from build123d import *

# Parameters (mm, degrees)
SKETCH_1_R          = 3
EXTRUDE_1_DEPTH     = 5
EXTRUDE_1_2_DEPTH   = 5
EXTRUDE_1_3_DEPTH   = 5
EXTRUDE_1_4_DEPTH   = 5
SKETCH_2_R          = 30
EXTRUDE_2_DEPTH     = 5
SKETCH_3_R          = 10.75
CUT_EXTRUDE_1_DEPTH = 5
SKETCH_4_R          = 17
SKETCH_4_R_2        = 15
CUT_EXTRUDE_3_DEPTH = 3


with BuildPart() as part:
    # Sketch 1 → Extrude 1 (new body)
    with BuildSketch(Plane.XY):
        with Locations((25, 0)):
            Circle(SKETCH_1_R)
    extrude(amount=-EXTRUDE_1_DEPTH)



with BuildPart() as body_2:
    # Sketch 1 → Extrude 1 2 (new body)
    with BuildSketch(Plane.XY):
        with Locations((0, -25)):
            Circle(SKETCH_1_R)
    extrude(amount=-EXTRUDE_1_2_DEPTH)


with BuildPart() as body_3:
    # Sketch 1 → Extrude 1 3 (new body)
    with BuildSketch(Plane.XY):
        with Locations((-25, 0)):
            Circle(SKETCH_1_R)
    extrude(amount=-EXTRUDE_1_3_DEPTH)


with BuildPart() as body_4:
    # Sketch 1 → Extrude 1 4 (new body)
    with BuildSketch(Plane.XY):
        with Locations((0, 25)):
            Circle(SKETCH_1_R)
    extrude(amount=-EXTRUDE_1_4_DEPTH)


with BuildPart() as part_1:
    add(part.part)

    add(body_2.part)  # Extrude 2 merges body 2

    add(body_3.part)  # Extrude 2 merges body 3

    add(body_4.part)  # Extrude 2 merges body 4
    # Sketch 2 → Extrude 2 (add)
    with BuildSketch(Plane(origin=(0, 0, -5), x_dir=(-1, 0, 0), z_dir=(0, 0, -1))):
        with Locations(Location((0, 0, 0), (0, 0, 180))):
            Circle(SKETCH_2_R)
    extrude(amount=EXTRUDE_2_DEPTH)

    # Sketch 3 → Cut-Extrude 1 (cut)
    with BuildSketch(Plane(origin=(0, 0, -10), x_dir=(-1, 0, 0), z_dir=(0, 0, -1))):
        Circle(SKETCH_3_R)
    extrude(amount=-CUT_EXTRUDE_1_DEPTH, mode=Mode.SUBTRACT)

    # Sketch 4 → Cut-Extrude 3 (cut)
    with BuildSketch(Plane(origin=(0, 0, -10), x_dir=(-1, 0, 0), z_dir=(0, 0, -1))):
        Circle(SKETCH_4_R)
        Circle(SKETCH_4_R_2, mode=Mode.SUBTRACT)
    extrude(amount=-CUT_EXTRUDE_3_DEPTH, mode=Mode.SUBTRACT)


solid = part_1.part
Model file for the job. Use its own axes, mm. A direction names the side the tool comes from. Give positions to 0.01 mm unless a question says otherwise; leave off trailing zeros. Loops run counter-clockwise (first coordinate to the right, second up) from the corner with the lowest first, then second, coordinate; pieces in that order, holes last.
1) Saw through at C-C (z = -3.75). Write the cut outline in (x, y), plus the area to 3 significant figures.
2) Saw through at B-B (y = -4.5). Write the cut outline in (x, z).
3) Tool access for faces 1 (the flat face through (25, 0, 0)), 2 (the flat face through (-6, -14, -7)), 3 (the flat face through (0, 13, -5)): list every direction of +Z, -Z, +X, -X, +Y, -Y with a clear straight run to the whole face (end or side of a thin tool).
4) Pull direction X, two halves, no side cores. Call faces 4 (the flat face through (13, 13, -10)), 5 (the cylindrical face through (16.128, -25.296, -7.465)), 6 (the cylindrical face through (-9.139, 14.334, -8.521)): +X half, -X half, draft (parallel to the pull), parting line (faces both ways), or undercut.
5) Saw through at A-A (x = 0). Write the cut outline in (y, z), plus the area to 4 significant figures.
6) Flat gauge pins, fed straight in: pin 1 Ø4 at (x, z) = (6.5, -4) entering from -Y; pin 2 Ø1.5 at (y, z) = (20, -7.5) entering from -X; pin 3 Ø1.5 at (x, y) = (9.5, 13) entering from -Z. Where does each tip first touch, or does it go through?
7) Saw through at D-D (y = 13). Write the cut outline in (x, z).
8) Wall check: line 1 (Y direction, x = 0, z = -8.15); line 2 (X direction, y = 3, z = -7.25); line 3 (Z direction, x = -20, y = 14). Give the ranges that are in metal, low to high.
Answer block:
1. outline: circle Ø6 at (-25, 0); circle Ø6 at (0, -25); circle Ø6 at (0, 25); circle Ø6 at (25, 0)
1. area: 113 mm2
2. outline: (-29.66, -10) - (-16.39, -10) - (-16.39, -7) - (-14.31, -7) - (-14.31, -10) - (-9.76, -10) - (-9.76, -5) - (-29.66, -5) - close; (9.76, -10) - (14.31, -10) - (14.31, -7) - (16.39, -7) - (16.39, -10) - (29.66, -10) - (29.66, -5) - (9.76, -5) - close
3. face 1: +Z, +X, -X, +Y, -Y
3. face 2: -Z
3. face 3: +Z
4. face 4: draft
4. face 5: parting line
4. face 6: undercut
5. outline: (-30, -10) - (-17, -10) - (-17, -7) - (-15, -7) - (-15, -10) - (-10.75, -10) - (-10.75, -5) - (-22, -5) - (-22, 0) - (-28, 0) - (-28, -5) - (-30, -5) - close; (10.75, -10) - (15, -10) - (15, -7) - (17, -7) - (17, -10) - (30, -10) - (30, -5) - (28, -5) - (28, 0) - (22, 0) - (22, -5) - (10.75, -5) - close
5. area: 240.5 mm2
6. pin 1: stops at y = -29.62
6. pin 2: stops at x = -23.01
6. pin 3: stops at z = -7
7. outline: (-27.04, -10) - (-10.95, -10) - (-10.95, -7) - (-7.48, -7) - (-7.48, -10) - (7.48, -10) - (7.48, -7) - (10.95, -7) - (10.95, -10) - (27.04, -10) - (27.04, -5) - (-27.04, -5) - close
8. line 1: y = -30 to -17, -15 to -10.75, 10.75 to 15, 17 to 30
8. line 2: x = -29.85 to -16.73, -14.7 to -10.32, 10.32 to 14.7, 16.73 to 29.85
8. line 3: z = -10 to -5
